Work out the finished part from the listing and answer in its coordinate system (mm). A direction names the side the tool comes from. Round coordinates to 2 decimals unless told otherwise and drop trailing zeros. Loops run counter-clockwise (first coordinate to the right, second up) from the corner with the lowest first, then second, coordinate; pieces in that order, holes last. Notation, with made-up numbers: (9, -4.5) - (47, -4.5) arc R27 cw to (47, 19.5) - close; hole circle Ø9 at (-4, 19.25). An arc over 180 degrees is marked (long way). Return JSON: item names as keys, results as strings.
from build123d import *

# Parameters (mm, degrees)
CROQUIS1_W              = 170
CROQUIS1_H              = 147
CROQUIS1_R              = 0.65
SALIENTE_EXTRUIR1_DEPTH = 15
CROQUIS2_R              = 6
CROQUIS2_R_2            = 2.75
CORTAR_EXTRUIR1_DEPTH   = 226.242091981
CROQUIS3_R              = 10
CORTAR_EXTRUIR2_DEPTH   = 4
CROQUIS5_R              = 2.5
CORTAR_EXTRUIR4_DEPTH   = 226.242091981
CROQUIS7_W              = 194.996484343
CROQUIS7_H              = 184.60954518
CORTAR_EXTRUIR6_DEPTH   = 226.242091981
CROQUIS8_R              = 2.5
SALIENTE_EXTRUIR2_DEPTH = 49
CROQUIS11_R             = 3.25
CROQUIS11_R_2           = 2.75
CORTAR_EXTRUIR9_DEPTH   = 20
CROQUIS12_R             = 1.997516107
CROQUIS12_R_2           = 2
CORTAR_EXTRUIR10_DEPTH  = 12
CROQUIS13_W             = 135.039321601
CROQUIS13_H             = 118.061076797
CORTAR_EXTRUIR11_DEPTH  = 40
CROQUIS14_W             = 119.536996173
CROQUIS14_H             = 17.5
CROQUIS14_W_2           = 122.159118923
CORTAR_EXTRUIR12_DEPTH  = 14
CROQUIS10_R             = 4.5
CORTAR_EXTRUIR8_DEPTH   = 6
CROQUIS15_R             = 3.89592378
CROQUIS15_R_2           = 2.9773148
SALIENTE_EXTRUIR3_DEPTH = 24
CORTAR_EXTRUIR13_START  = -9
CORTAR_EXTRUIR13_DEPTH  = 9
CROQUIS17_R             = 3
CROQUIS17_R_2           = 4
CORTAR_EXTRUIR14_DEPTH  = 24


with BuildPart() as part:
    # Croquis1 → Saliente-Extruir1 (new body)
    with BuildSketch(Plane.XY):
        with Locations((85, 73.5)):
            Rectangle(CROQUIS1_W, CROQUIS1_H)
        with Locations((102.354765644, 71.387865203)):
            Circle(CROQUIS1_R, mode=Mode.SUBTRACT)
        with Locations((68.004765644, 60.387865203)):
            Circle(CROQUIS1_R, mode=Mode.SUBTRACT)
        with Locations((68.004765644, 58.237865203)):
            Circle(CROQUIS1_R, mode=Mode.SUBTRACT)
        with Locations((70.104765644, 64.887865203)):
            Circle(CROQUIS1_R, mode=Mode.SUBTRACT)
        with Locations((70.104765644, 67.037865203)):
            Circle(CROQUIS1_R, mode=Mode.SUBTRACT)
        with Locations((100.854765644, 69.887865203)):
            Circle(CROQUIS1_R, mode=Mode.SUBTRACT)
    extrude(amount=SALIENTE_EXTRUIR1_DEPTH)

    # Croquis2 → Cortar-Extruir1 (cut, through all)
    with BuildSketch(Plane(origin=(0, 0, 0), x_dir=(-1, 0, 0), z_dir=(0, 0, -1))):
        with Locations((-52.054764009, 86.037865203)):
            Circle(CROQUIS2_R)
        with Locations((-117.054764009, 86.037865203)):
            Circle(CROQUIS2_R)
        with Locations((-117.054764009, 41.037865203)):
            Circle(CROQUIS2_R)
        with Locations((-52.054764009, 41.037865203)):
            Circle(CROQUIS2_R)
        with Locations((-117.054764009, 63.537865203)):
            Circle(CROQUIS2_R_2)
        with Locations((-52.054764009, 63.537865203)):
            Circle(CROQUIS2_R_2)
        with Locations((-84.554764009, 86.037865203)):
            Circle(CROQUIS2_R_2)
        with Locations((-84.554764009, 41.037865203)):
            Circle(CROQUIS2_R_2)
    extrude(amount=-CORTAR_EXTRUIR1_DEPTH, mode=Mode.SUBTRACT)

    # Croquis3 → Cortar-Extruir2 (cut)
    with BuildSketch(Plane(origin=(0, 0, 0), x_dir=(-1, 0, 0), z_dir=(0, 0, -1))):
        with Locations((-52.054764009, 86.037865203)):
            Circle(CROQUIS3_R)
        with Locations((-117.054764009, 86.037865203)):
            Circle(CROQUIS3_R)
        with Locations((-117.054764009, 41.037865203)):
            Circle(CROQUIS3_R)
        with Locations((-52.054764009, 41.037865203)):
            Circle(CROQUIS3_R)
    extrude(amount=-CORTAR_EXTRUIR2_DEPTH, mode=Mode.SUBTRACT)

    # Croquis5 → Cortar-Extruir4 (cut, through all)
    with BuildSketch(Plane(origin=(0, 0, 0), x_dir=(-1, 0, 0), z_dir=(0, 0, -1))):
        with Locations((-84.554764009, 111.037865203)):
            Circle(CROQUIS5_R)
        with Locations((-44.554764009, 111.037865203)):
            Circle(CROQUIS5_R)
        with Locations((-129.51388638, 111.061182682)):
            Circle(CROQUIS5_R)
        with Locations(Location((-129.51388638, 16.014547725, 0), (0, 0, 180))):
            Circle(CROQUIS5_R)
        with Locations(Location((-39.554764009, 16.037865203, 0), (0, 0, 180))):
            Circle(CROQUIS5_R)
        with Locations(Location((-84.554764009, 16.037865203, 0), (0, 0, 180))):
            Circle(CROQUIS5_R)
    extrude(amount=-CORTAR_EXTRUIR4_DEPTH, mode=Mode.SUBTRACT)

    # Croquis7 → Cortar-Extruir6 (cut, through all)
    with BuildSketch(Plane(origin=(0, 0, 0), x_dir=(-1, 0, 0), z_dir=(0, 0, -1))):
        with Locations((-84.554764009, 63.537865203)):
            Rectangle(CROQUIS7_W, CROQUIS7_H)
        with BuildLine():
            Line((-134.554764009, 8.537865203), (-34.554764009, 8.537865203))
            ThreePointArc((-34.554764009, 8.537865203), (-31.019230103, 10.002331297), (-29.554764009, 13.537865203))
            Line((-29.554764009, 13.537865203), (-29.554764009, 113.537865203))
            ThreePointArc((-29.554764009, 113.537865203), (-31.019230103, 117.073399109), (-34.554764009, 118.537865203))
            Line((-34.554764009, 118.537865203), (-134.554764009, 118.537865203))
            ThreePointArc((-134.554764009, 118.537865203), (-138.090297915, 117.073399109), (-139.554764009, 113.537865203))
            Line((-139.554764009, 113.537865203), (-139.554764009, 13.537865203))
            ThreePointArc((-139.554764009, 13.537865203), (-138.090297915, 10.002331297), (-134.554764009, 8.537865203))
        make_face(mode=Mode.SUBTRACT)
    extrude(amount=-CORTAR_EXTRUIR6_DEPTH, mode=Mode.SUBTRACT)

    # Croquis8 → Saliente-Extruir2 (add)
    with BuildSketch(Plane.XY.offset(15)):
        with BuildLine():
            Line((29.554764009, 113.537865203), (29.554764009, 13.537865203))
            ThreePointArc((29.554764009, 13.537865203), (31.019230103, 10.002331297), (34.554764009, 8.537865203))
            Line((34.554764009, 8.537865203), (134.554764009, 8.537865203))
            ThreePointArc((134.554764009, 8.537865203), (138.090297915, 10.002331297), (139.554764009, 13.537865203))
            Line((139.554764009, 13.537865203), (139.554764009, 113.537865203))
            ThreePointArc((139.554764009, 113.537865203), (138.090297915, 117.073399109), (134.554764009, 118.537865203))
            Line((134.554764009, 118.537865203), (34.554764009, 118.537865203))
            ThreePointArc((34.554764009, 118.537865203), (31.019230103, 117.073399109), (29.554764009, 113.537865203))
        make_face()
        with Locations(Location((44.554764009, 111.037865203, 0), (0, 0, 180))):
            Circle(CROQUIS8_R, mode=Mode.SUBTRACT)
        with Locations(Location((84.554764009, 111.037865203, 0), (0, 0, 180))):
            Circle(CROQUIS8_R, mode=Mode.SUBTRACT)
        with Locations(Location((129.51388638, 111.061182682, 0), (0, 0, 180))):
            Circle(CROQUIS8_R, mode=Mode.SUBTRACT)
        with Locations((129.51388638, 16.014547725)):
            Circle(CROQUIS8_R, mode=Mode.SUBTRACT)
        with Locations((84.554764009, 16.037865203)):
            Circle(CROQUIS8_R, mode=Mode.SUBTRACT)
        with Locations((39.554764009, 16.037865203)):
            Circle(CROQUIS8_R, mode=Mode.SUBTRACT)
        with BuildLine():
            Line((47.558208504, 31.037865203), (121.558208504, 31.037865203))
            ThreePointArc((121.558208504, 31.037865203), (124.386635629, 32.209438078), (125.558208504, 35.037865203))
            Line((125.558208504, 35.037865203), (125.558208504, 92.037865203))
            ThreePointArc((125.558208504, 92.037865203), (124.386635629, 94.866292328), (121.558208504, 96.037865203))
            Line((121.558208504, 96.037865203), (47.558208504, 96.037865203))
            ThreePointArc((47.558208504, 96.037865203), (44.72978138, 94.866292328), (43.558208504, 92.037865203))
            Line((43.558208504, 92.037865203), (43.558208504, 35.037865203))
            ThreePointArc((43.558208504, 35.037865203), (44.72978138, 32.209438078), (47.558208504, 31.037865203))
        make_face(mode=Mode.SUBTRACT)
    extrude(amount=SALIENTE_EXTRUIR2_DEPTH)

    # Croquis11 → Cortar-Extruir9 (cut)
    with BuildSketch(Plane(origin=(0, 0, 0), x_dir=(-1, 0, 0), z_dir=(0, 0, -1))):
        with Locations((-41.554764009, 63.537865203)):
            Circle(CROQUIS11_R)
        with Locations((-135.554764009, 63.537865203)):
            Circle(CROQUIS11_R_2)
    extrude(amount=-CORTAR_EXTRUIR9_DEPTH, mode=Mode.SUBTRACT)

    # Croquis12 → Cortar-Extruir10 (cut)
    with BuildSketch(Plane(origin=(0, 0, 0), x_dir=(-1, 0, 0), z_dir=(0, 0, -1))):
        with Locations((-36.554764009, 94.037865203)):
            Circle(CROQUIS12_R)
        with Locations((-36.554764009, 33.037865203)):
            Circle(CROQUIS12_R_2)
        with Locations((-132.554764009, 33.037865203)):
            Circle(CROQUIS12_R_2)
        with Locations((-132.554764009, 94.037865203)):
            Circle(CROQUIS12_R_2)
    extrude(amount=-CORTAR_EXTRUIR10_DEPTH, mode=Mode.SUBTRACT)

    # Croquis13 → Cortar-Extruir11 (cut)
    with BuildSketch(Plane.XY.offset(64)):
        with Locations((90.028445249, 63.21009986)):
            Rectangle(CROQUIS13_W, CROQUIS13_H)
    extrude(amount=-CORTAR_EXTRUIR11_DEPTH, mode=Mode.SUBTRACT)

    # Croquis14 → Cortar-Extruir12 (cut)
    with BuildSketch(Plane(origin=(0, 0, 0), x_dir=(-1, 0, 0), z_dir=(0, 0, -1))):
        with Locations((-79.786265922, 109.787865203)):
            Rectangle(CROQUIS14_W, CROQUIS14_H)
        with Locations((-78.475204547, 17.287865203)):
            Rectangle(CROQUIS14_W_2, CROQUIS14_H)
    extrude(amount=-CORTAR_EXTRUIR12_DEPTH, mode=Mode.SUBTRACT)

    # Croquis10 → Cortar-Extruir8 (cut)
    with BuildSketch(Plane(origin=(0, 0, 14), x_dir=(-1, 0, 0), z_dir=(0, 0, -1))):
        with Locations((-44.554764009, 111.037865203)):
            Circle(CROQUIS10_R)
        with Locations((-84.554764009, 111.037865203)):
            Circle(CROQUIS10_R)
        with Locations((-129.51388638, 111.061182682)):
            Circle(CROQUIS10_R)
        with Locations((-129.554764009, 16.037865203)):
            Circle(CROQUIS10_R)
        with Locations((-84.554764009, 16.037865203)):
            Circle(CROQUIS10_R)
        with Locations((-39.554764009, 16.037865203)):
            Circle(CROQUIS10_R)
    extrude(amount=-CORTAR_EXTRUIR8_DEPTH, mode=Mode.SUBTRACT)

    # Croquis15 → Saliente-Extruir3 (add)
    with BuildSketch(Plane(origin=(0, 0, 0), x_dir=(-1, 0, 0), z_dir=(0, 0, -1))):
        with Locations((-41.554764009, 63.537865203)):
            Circle(CROQUIS15_R)
        with Locations((-135.554764009, 63.537865203)):
            Circle(CROQUIS15_R_2)
    extrude(amount=-SALIENTE_EXTRUIR3_DEPTH)

    # Croquis16 → Cortar-Extruir13 (cut)
    with BuildSketch(Plane.XY.offset(24).offset(CORTAR_EXTRUIR13_START)):
        with BuildLine():
            Line((43.558208504, 66.879187135), (43.558208504, 60.196543272))
            ThreePointArc((43.558208504, 60.196543272), (45.450687788, 63.537865203), (43.558208504, 66.879187135))
        make_face()
    extrude(amount=CORTAR_EXTRUIR13_DEPTH, mode=Mode.SUBTRACT)

    # Croquis17 → Cortar-Extruir14 (cut)
    with BuildSketch(Plane(origin=(0, 0, 0), x_dir=(-1, 0, 0), z_dir=(0, 0, -1))):
        with Locations((-37.65059727, 64.010566888)):
            Circle(CROQUIS17_R)
        with Locations((-131.65059727, 64.010566888)):
            Circle(CROQUIS17_R_2)
    extrude(amount=-CORTAR_EXTRUIR14_DEPTH, mode=Mode.SUBTRACT)


solid = part.part
1) Flat-ended cylindrical pins translate along their axes: pin 1 (10 mm diameter, centred on x = 53.5, y = 42, fed in from -Z); pin 2 (2 mm diameter, centred on x = 102.35, y = 71.39, fed in from +Z); pin 3 (5 mm diameter, centred on x = 41.5, z = 9.5, fed in from -Y); pin 4 (3 mm diameter, centred on x = 84.55, y = 16.04, fed in from +Z). Find the tip coordinate at first contact, or state that the pin passes through.
Verdict:
{"pin 1": "stops at z = 4", "pin 2": "stops at z = 15", "pin 3": "stops at y = 26.04", "pin 4": "passes through"}
2) Section A-A (x = 78) is taken. Give the vertices of the cut face in (y, z).
Verdict:
{"outline": "(8.54, 14) - (26.04, 14) - (26.04, 0) - (101.04, 0) - (101.04, 14) - (118.54, 14) - (118.54, 24) - (96.04, 24) - (96.04, 15) - (31.04, 15) - (31.04, 24) - (8.54, 24) - close"}
3) Section D-D (y = 49) is taken. Give the vertices of the cut face in (x, z), and give its area (3 significant figures).
Verdict:
{"outline": "(29.55, 0) - (46, 0) - (46, 4) - (58.1, 4) - (58.1, 0) - (111, 0) - (111, 4) - (123.1, 4) - (123.1, 0) - (139.55, 0) - (139.55, 24) - (125.56, 24) - (125.56, 15) - (43.56, 15) - (43.56, 24) - (29.55, 24) - close", "area": "1,810 mm2"}
4) A tool of negligible diameter and unlimited length cuts with its end or side. For faces 4 (the flat face through (85, 101.038, 7)), 5 (the flat face through (84, 64, 15)), 6 (the flat face through (117.2, 34.5, 4)), from which of +Z, -Z, +X, -X, +Y, -Y can it reach the whole face along a straight path? Write none if from no direction.
Verdict:
{"face 4": "-Z, +X, -X, +Y", "face 5": "+Z", "face 6": "-Z"}
5) Find the intervals of material crossed by L1, parallel to Y at x = 116, z = 15.25; L2, parallel to X at y = 84, z = 18.25; L3, parallel to Y at x = 47.5, z = 2.75, in increasing order.
Verdict:
{"L1": "y = 8.54 to 31.04, 96.04 to 118.54", "L2": "x = 29.55 to 43.56, 125.56 to 139.55", "L3": "y = 26.04 to 32.14, 49.94 to 77.14, 94.94 to 101.04"}
6) Section B-B (z = 8) is taken. Count the separate pieces of the cut face and the enclosed holes in it, and give its area (3 significant figures).
Verdict:
{"separate pieces": "1", "enclosed holes": "20", "area": "7,570 mm2"}
7) Determine the mould class of faces 1 (the flat face through (85, 96.038, 19)), 2 (the flat face through (139.555, 63, 12)), 3 (the flat face through (84, 8.538, 19)) for opening direction X: pulls with the +X half, pulls with the -X half, needs draft (parallel to the pull), parting line crosses it, or undercut.
Verdict:
{"face 1": "undercut", "face 2": "pulls with the +X half", "face 3": "needs draft"}
